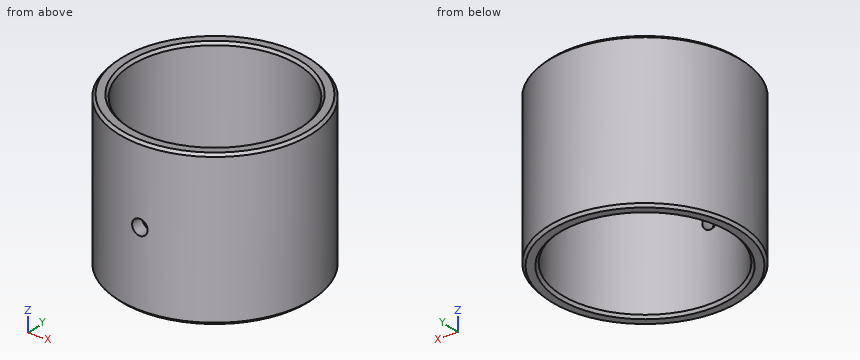
```python
from build123d import *

# Parameters (mm, degrees)
SKETCH_1_R          = 37.5
SKETCH_1_R_2        = 32.5
EXTRUDE_1_DEPTH     = 30
CHAMFER_1_SIZE      = 1
SKETCH_2_R          = 3
CUT_EXTRUDE_1_DEPTH = 61.930288035


with BuildPart() as part:
    # 草图1 → 凸台-拉伸1 (new, symmetric)
    with BuildSketch(Plane.XY):
        Circle(SKETCH_1_R)
        Circle(SKETCH_1_R_2, mode=Mode.SUBTRACT)
    extrude(amount=EXTRUDE_1_DEPTH, both=True)

    # 倒角1
    chamfer_1_edges = [part.edges().sort_by_distance(p)[0] for p in [
        (-37.5, 0, -30),
        (-37.5, 0, 30),
        (-32.5, 0, -30),
        (-32.5, 0, 30),
    ]]
    chamfer(chamfer_1_edges, length=CHAMFER_1_SIZE)

    # 草图2 → 切除-拉伸1 (cut, through all)
    with BuildSketch(Plane(origin=(0, 0, 0), x_dir=(1, 0, 0), z_dir=(0, 1, 0))):
        with Locations(Location((0, 0, 0), (0, 0, 270))):
            Circle(SKETCH_2_R)
    extrude(amount=-CUT_EXTRUDE_1_DEPTH, mode=Mode.SUBTRACT)


solid = part.part
```
The listing builds one solid part. Answer for the finished solid, in the listing's coordinates (mm). Coordinates: 2 decimals unless noted, no trailing zeros. Order: outer loops, then holes, each group sorted by start corner. A loop starts at its lowest first (then second) coordinate and runs counter-clockwise, first axis right, second up. Notation, with made-up numbers: M -6.5,-21 L 6.5,-21 A20 cw 6.5,7 Z; hole C -19,-34.5 d3. An arc over 180 degrees is marked long. Answer as a JSON object with one key per item and string values. Group by question number.
1. Section C-C on z = 5 is taken. Write down the section's boundary in (x, y).
2. Section B-B on x = 0 is taken. Write down the section's boundary in (y, z).
3. Straight lines are drawn through the part: line 1 (Y direction, x = 0, z = 15.5); line 2 (Y direction, x = 0, z = 2); line 3 (Z direction, x = 0, y = -34.5). For each, find the intervals that lie inside material, in ascending order.
4. Section A-A on y = 0 is taken. Write down the section's boundary in (x, z), then the cut area to 3 significant figures.
5. Flat-ended cylindrical pins translate along their axes: P1, Ø6, axis at y = 4, z = -11.5, coming from the -X side; P2, Ø4, axis at x = -6.5, z = -14.5, coming from the -Y side; P3, Ø8, axis at x = -4.5, z = 21.5, coming from the -Y side. Find the tip coordinate at first contact, or state that the pin passes through.
Values follow:
{
 "1": {"outline": "C 0,0 d75; hole C 0,0 d65"},
 "2": {"outline": "M -37.5,-29 L -36.5,-30 L -33.5,-30 L -32.5,-29 L -32.5,-3 L -37.5,-3 Z; M -37.5,3 L -32.5,3 L -32.5,29 L -33.5,30 L -36.5,30 L -37.5,29 Z; M 32.5,-29 L 33.5,-30 L 36.5,-30 L 37.5,-29 L 37.5,29 L 36.5,30 L 33.5,30 L 32.5,29 Z"},
 "3": {"line 1": "-37.5 to -32.5, 32.5 to 37.5", "line 2": "32.5 to 37.5", "line 3": "-30 to -3, 3 to 30"},
 "4": {"outline": "M -37.5,-29 L -36.5,-30 L -33.5,-30 L -32.5,-29 L -32.5,29 L -33.5,30 L -36.5,30 L -37.5,29 Z; M 32.5,-29 L 33.5,-30 L 36.5,-30 L 37.5,-29 L 37.5,29 L 36.5,30 L 33.5,30 L 32.5,29 Z", "area": "596 mm2"},
 "5": {"P1": "x = -37.49", "P2": "y = -37.23", "P3": "y = -37.5"}
}
